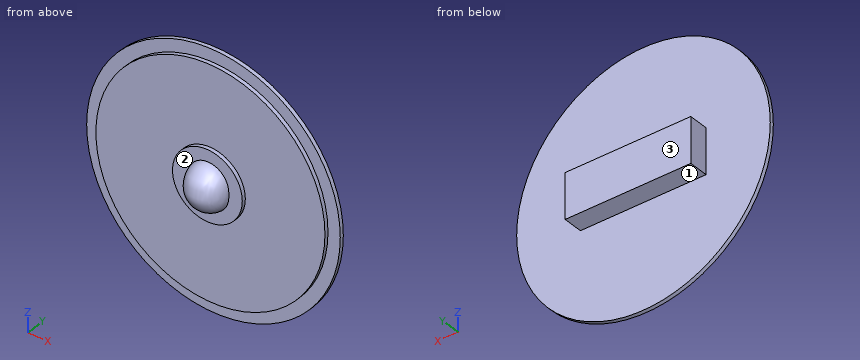
```python
from build123d import *

# Parameters (mm, degrees)
F0_R     = 64.6501661092
F1_DEPTH = 2
F2_R     = 58.3906785059
F3_DEPTH = 2
F6_W     = 64.0570893884
F6_H     = 23.0703689158
F7_DEPTH = 10
F8_R     = 17.7936347266
F9_DEPTH = 2


with BuildPart() as f1:
    # F0 (on Front) → F1 (new body)
    with BuildSketch(Plane.XZ):
        Circle(F0_R)
    extrude(amount=F1_DEPTH)

    # F2 (on face) → F3 (join)
    with BuildSketch(Plane.XZ.offset(2)):
        Circle(F2_R)
    extrude(amount=F3_DEPTH)

    # F4 (on Top) → F5 (revolve)
    with BuildSketch(Plane.XY):
        with BuildLine():
            Line((10.7988948002, -3.8041563239), (-9.8171774298, -4.295015242))
            ThreePointArc((-9.8171774298, -4.295015242), (0.7757822444, -16.0163739159), (10.7988948002, -3.8041563239))
        make_face()
    revolve(axis=Axis((0.4908586852, -4.0495857829, 0), (0.9997166737, 0.0238027806, 0)))

    # F6 (on face) → F7 (join)
    with BuildSketch(Plane(origin=(0, 0, 0), x_dir=(-1, 0, 0), z_dir=(0, 1, 0))):
        with Locations((-0.1227147877, -0.1227147877)):
            Rectangle(F6_W, F6_H)
    extrude(amount=F7_DEPTH)

    # F8 (on face) → F9 (join)
    with BuildSketch(Plane.XZ.offset(4)):
        Circle(F8_R)
    extrude(amount=F9_DEPTH)


solid = f1.part
```
Check sheet for the modelled part. Datum: model origin and axes. Units: mm. Face numbers are marked on the shaded views. A direction names the side the tool comes from. Give positions to 0.01 mm unless a question says otherwise; leave off trailing zeros. Loops run counter-clockwise (first coordinate to the right, second up) from the corner with the lowest first, then second, coordinate; pieces in that order, holes last. Notation, with made-up numbers: M -5,72.5 L 15,72.5 A37 ccw 15,109.5 Z; hole C 42.5,50 d4. An arc over 180 degrees is marked long. Answer in a Markdown table with one row per item.
1) Depth check by flat-ended pin: pin 1 (8 mm diameter, centred on x = 11, y = 6.5, fed in from +Z); pin 2 (12 mm diameter, centred on x = 14.5, z = -26, fed in from -Y); pin 3 (6 mm diameter, centred on x = -49.5, z = 43, fed in from -Y). Enter the tip coordinate at first touch or a pass-through.
Solutions:
| item | result |
|---|---|
| pin 1 | stops at z = 11.41 |
| pin 2 | stops at y = -4 |
| pin 3 | stops at y = -2 |
2) Thickness scan on line 1 (X direction, y = 2, z = 9); line 2 (Y direction, x = 50, z = -1.5); line 3 (Y direction, x = 29, z = -55). Record the ranges inside material, lowest first.
Solutions:
| item | result |
|---|---|
| line 1 | x = -31.91 to 32.15 |
| line 2 | y = -4 to 0 |
| line 3 | y = -2 to 0 |
3) Cross-section at A-A (z = -36). Enter the section's corners in (x, y), plus the area to 3 significant figures.
Solutions:
| item | result |
|---|---|
| outline | M -53.7,-2 L -45.97,-2 L -45.97,-4 L 45.97,-4 L 45.97,-2 L 53.7,-2 L 53.7,0 L -53.7,0 Z |
| area | 399 mm^2 |
4) Cross-section at B-B (y = 4). Enter the section's corners in (x, z), plus the area to 3 significant figures.
Solutions:
| item | result |
|---|---|
| outline | M -31.91,-11.66 L 32.15,-11.66 L 32.15,11.41 L -31.91,11.41 Z |
| area | 1,480 mm^2 |
5) Tool access check on the marked faces 1, 2 and 3. Record the directions out of +Z, -Z, +X, -X, +Y, -Y that give a thin tool (end or side, any length) a straight path to the whole face; none if there is none.
Solutions:
| item | result |
|---|---|
| face 1 | -Z, +X, -X, +Y |
| face 2 | -Y |
| face 3 | +Z, -Z, +X, -X, +Y |
6) Cross-section at C-C (x = -51). Enter the section's corners in (y, z), plus the area to 3 significant figures.
Solutions:
| item | result |
|---|---|
| outline | M -4,-28.43 L -2,-28.43 L -2,-39.73 L 0,-39.73 L 0,39.73 L -2,39.73 L -2,28.43 L -4,28.43 Z |
| area | 273 mm^2 |
